Can you work these out from the model? Positions are in its coordinate system, mm. Round coordinates to 2 decimals unless told otherwise and drop trailing zeros. Write each loop counter-clockwise with the first axis right and the second up, starting at its lowest first coordinate (ties: lowest second). Pieces come first, ordered by that corner, then holes.
Q1. If we section it at C-C (x = -1): Please give me the cut outline in (y, z).
Q2. If we section it at B-B (x = -5.5): Please give me the cut outline in (y, z), plus the area to 3 significant figures.
Q3. I'm going to push flat-ended pins straight in: pin 1 Ø6 at (y, z) = (-7, 68.5) entering from +X; pin 2 Ø5 at (x, z) = (6, 31.5) entering from -Y; pin 3 Ø2 at (x, z) = (7.5, 54) entering from +Y; pin 4 Ø8 at (y, z) = (1, 70.5) entering from -X. Where does each tip first touch, or does it pass through?
Q4. If we section it at A-A (y = 1.25): Please give me the cut outline in (x, z).
Q5. If we section it at D-D (z = 13): Please give me the cut outline in (x, y) (3 decimals), plus the area to 3 significant figures.
Q6. We'd pull the mould along Y, two halves only. Please class faces 1 (the cylindrical face through (11.45, -4.75, 41.85)), 2 (the flat face through (-5.45, -10.96, 82.55)), 3 (the cylindrical face through (11.51, 3.62, 41.85)): +Y half, -Y half, draft (parallel to the pull), parting line (faces both ways), or undercut.
Q7. Please list where these lines run through material, in increasing order: line 1 along Y through (x, z) = (0, 21) (3 decimals); line 2 along Y through (x, z) = (-2, 4); line 3 along X through (y, z) = (-1, 37).
from build123d import *

# Parameters (mm, degrees)
F0_W      = 0.3302
F0_H      = 82.55
F3_DEPTH  = 12.3962
F7_DEPTH  = 1.7554578348
F10_DEPTH = 1.7554578348


with BuildPart() as f1:
    # F0 (on Front) → F1 (revolve)
    with BuildSketch(Plane.XZ):
        with Locations((12.2301, 41.275)):
            Rectangle(F0_W, F0_H)
    revolve(axis=Axis((0, 0, 41.275), (0, 0, 1)))

    # F2 (on Front) → F3 (cut, through all)
    with BuildSketch(Plane.XZ):
        with BuildLine():
            ThreePointArc((0, 60.325), (-3.175, 57.15), (0, 53.975))
            Line((0, 53.975), (0, 60.325))
        make_face()
        with BuildLine():
            Line((0, 60.325), (0, 53.975))
            ThreePointArc((0, 53.975), (2.2450640303, 54.9049359697), (3.175, 57.15))
            ThreePointArc((3.175, 57.15), (2.2450640303, 59.3950640303), (0, 60.325))
        make_face()
    extrude(amount=F3_DEPTH, mode=Mode.SUBTRACT)

    # F6 (on line) → F7 (cut, up to face)
    with BuildSketch(Plane(origin=(10.734558085, 6.1976, 0), x_dir=(-0.5, 0.8660254038, 0), z_dir=(0.8660254038, 0.5, 0))):
        with BuildLine():
            ThreePointArc((0, 60.325), (-3.175, 57.15), (0, 53.975))
            Line((0, 53.975), (0, 60.325))
        make_face()
        with BuildLine():
            Line((0, 60.325), (0, 53.975))
            ThreePointArc((0, 53.975), (2.2450640303, 54.9049359697), (3.175, 57.15))
            ThreePointArc((3.175, 57.15), (2.2450640303, 59.3950640303), (0, 60.325))
        make_face()
    extrude(amount=-F7_DEPTH, mode=Mode.SUBTRACT)

    # F9 (on line) → F10 (cut, up to face)
    with BuildSketch(Plane(origin=(-10.734558085, 6.1976, 0), x_dir=(-0.5, -0.8660254038, 0), z_dir=(-0.8660254038, 0.5, 0))):
        with BuildLine():
            ThreePointArc((0, 60.325), (-3.175, 57.15), (0, 53.975))
            Line((0, 53.975), (0, 60.325))
        make_face()
        with BuildLine():
            Line((0, 60.325), (0, 53.975))
            ThreePointArc((0, 53.975), (2.2450640303, 54.9049359697), (3.175, 57.15))
            ThreePointArc((3.175, 57.15), (2.2450640303, 59.3950640303), (0, 60.325))
        make_face()
    extrude(amount=-F10_DEPTH, mode=Mode.SUBTRACT)


solid = f1.part
A:
1. outline: (-12.35, 0) - (-12.02, 0) - (-12.02, 54.14) - (-12.35, 54.14) - close; (-12.35, 60.16) - (-12.02, 60.16) - (-12.02, 82.55) - (-12.35, 82.55) - close; (12.02, 0) - (12.35, 0) - (12.35, 82.55) - (12.02, 82.55) - close
2. outline: (-11.11, 0) - (-10.74, 0) - (-10.74, 82.55) - (-11.11, 82.55) - close; (10.74, 0) - (11.11, 0) - (11.11, 82.55) - (10.74, 82.55) - close
2. area: 61.0 mm2
3. pin 1: stops at x = 11.73
3. pin 2: stops at y = -11.89
3. pin 3: stops at y = 10.55
3. pin 4: stops at x = -12.4
4. outline: (-12.33, 0) - (-12, 0) - (-12, 82.55) - (-12.33, 82.55) - close; (12, 0) - (12.33, 0) - (12.33, 82.55) - (12, 82.55) - close
5. outline: circle Ø24.79 at (0, 0); hole circle Ø24.13 at (0, 0)
5. area: 25.4 mm2
6. face 1: parting line
6. face 2: draft
6. face 3: undercut
7. line 1: y = -12.395 to -12.065, 12.065 to 12.395
7. line 2: y = -12.23 to -11.9, 11.9 to 12.23
7. line 3: x = -12.35 to -12.02, 12.02 to 12.35
